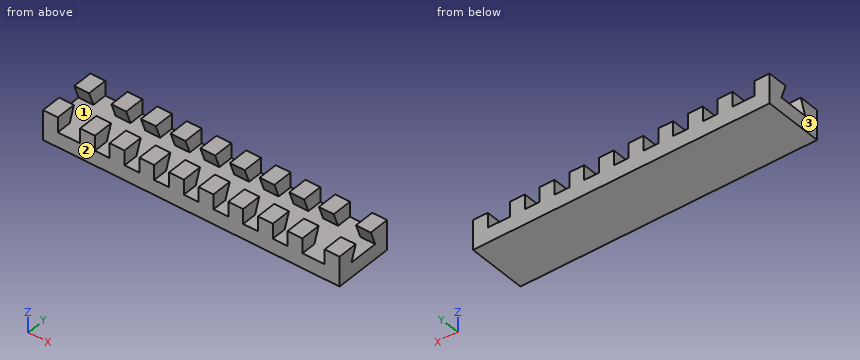
from build123d import *

# Parameters (mm, degrees)
F0_W     = 100
F0_H     = 20
F1_DEPTH = 10
F3_DEPTH = 100.001
F4_W     = 7.5
F4_H     = 5
F4_W_2   = 5
F5_DEPTH = 20.001


with BuildPart() as f1:
    # F0 (on Top) → F1 (new body)
    with BuildSketch(Plane.XY):
        Rectangle(F0_W, F0_H)
    extrude(amount=F1_DEPTH)

    # F2 (on face) → F3 (cut, through all)
    with BuildSketch(Plane.YZ.offset(50)):
        Polygon((3.180149, 10), (-3.180149, 10), (-5, 5), (5, 5), align=None)
    extrude(amount=-F3_DEPTH, mode=Mode.SUBTRACT)

    # F4 (on face) → F5 (cut, through all)
    with BuildSketch(Plane.XZ.offset(10)):
        with Locations((-41.25, 7.5)):
            Rectangle(F4_W, F4_H)
        with Locations((-30, 7.5)):
            Rectangle(F4_W_2, F4_H)
        with Locations((-20, 7.5)):
            Rectangle(F4_W_2, F4_H)
        with Locations((-10, 7.5)):
            Rectangle(F4_W_2, F4_H)
        with Locations((0, 7.5)):
            Rectangle(F4_W_2, F4_H)
        with Locations((10, 7.5)):
            Rectangle(F4_W_2, F4_H)
        with Locations((20, 7.5)):
            Rectangle(F4_W_2, F4_H)
        with Locations((30, 7.5)):
            Rectangle(F4_W_2, F4_H)
        with Locations((41.25, 7.5)):
            Rectangle(F4_W, F4_H)
    extrude(amount=-F5_DEPTH, mode=Mode.SUBTRACT)


solid = f1.part
Geometry: final body of the model. Coordinates: model frame, mm. Face numbers are marked on the shaded views. Give positions to 0.01 mm unless a question says otherwise; leave off trailing zeros. Order: outer loops, then holes, each group sorted by start corner. A loop starts at its lowest first (then second) coordinate and runs counter-clockwise, first axis right, second up. Notation, with made-up numbers: (26, 73) -> (61, 73) arc R25 ccw to (61, 85) -> close; hole circle Ø8 at (60.5, -36.75). An arc over 180 degrees is marked (long way). Answer as a JSON object with one key per item and string values.
Q1. Section B-B (z = 7). State how many separate pieces and enclosed holes the cut face has, plus the area to 3 significant figures.
Entries:
{"separate pieces": "20", "enclosed holes": "0", "area": "573 mm^2"}
Q2. Section D-D (x = 43.5). Output: boundary loops of the cut face in (y, z).
Entries:
{"outline": "(-10, 0) -> (10, 0) -> (10, 5) -> (-10, 5) -> close"}
Q3. Section C-C (y = -2). Output: boundary loops of the cut face in (x, z).
Entries:
{"outline": "(-50, 0) -> (50, 0) -> (50, 5) -> (-50, 5) -> close"}
Q4. Section A-A (x = 14). Output: boundary loops of the cut face in (y, z), plus the area to 3 significant figures.
Entries:
{"outline": "(-10, 0) -> (10, 0) -> (10, 10) -> (3.18, 10) -> (5, 5) -> (-5, 5) -> (-3.18, 10) -> (-10, 10) -> close", "area": "159 mm^2"}
Q5. Draft query along X for the marked faces 1, 2 and 3. Return one class per face: released by +X, released by -X, zero draft, split by the parting line, or undercut.
Entries:
{"face 1": "undercut", "face 2": "zero draft", "face 3": "released by -X"}
Q6. First-contact query: pin 1 (4 mm diameter, centred on x = -19, z = 9, fed in from +Y). Flat tip, straight axial feed; report the tip coordinate or a pass-through.
Entries:
{"pin 1": "stops at y = 10"}
Q7. Material intervals for probe 1 along Z at (x, y) = (-16, 2); probe 2 along Y at (x, z) = (35, 8.25); probe 3 along Y at (x, z) = (-14, 6), sorted ascending.
Entries:
{"probe 1": "z = 0 to 5", "probe 2": "y = -10 to -3.82, 3.82 to 10", "probe 3": "y = -10 to -4.64, 4.64 to 10"}
